from build123d import *

# Parameters (mm, degrees)
F0_R     = 11.509137
F1_DEPTH = 25.4
F2_DEPTH = 50.8


with BuildPart() as f1:
    # F0 (on Front) → F1 (new body)
    with BuildSketch(Plane.XZ):
        with BuildLine():
            ThreePointArc((-23.485197, 0), (0, -23.485197), (23.485197, 0))
            ThreePointArc((23.485197, 0), (0, 23.485197), (-23.485197, 0))
        make_face()
        Circle(F0_R, mode=Mode.SUBTRACT)
        with BuildLine():
            ThreePointArc((-23.485197, 0), (0, 23.485197), (23.485197, 0))
            Line((23.485197, 0), (23.485197, 74.391678))
            ThreePointArc((23.485197, 74.391678), (0, 50.906481), (-23.485197, 74.391678))
            Line((-23.485197, 74.391678), (-23.485197, 0))
        make_face()
        with BuildLine():
            ThreePointArc((-23.485197, 74.391678), (0, 50.906481), (23.485197, 74.391678))
            ThreePointArc((23.485197, 74.391678), (0, 97.876875), (-23.485197, 74.391678))
        make_face()
        with Locations((0, 74.391678)):
            Circle(F0_R, mode=Mode.SUBTRACT)
    extrude(amount=F1_DEPTH)

    # F0 (on Front) → F2 (join)
    with BuildSketch(Plane.XZ):
        with BuildLine():
            ThreePointArc((-23.485197, 0), (0, -23.485197), (23.485197, 0))
            ThreePointArc((23.485197, 0), (0, 23.485197), (-23.485197, 0))
        make_face()
        Circle(F0_R, mode=Mode.SUBTRACT)
    extrude(amount=-F2_DEPTH)

    # F3: F1 across face


with BuildPart() as f1_1:
    add(f1.part)
    add(f1.part.mirror(Plane(origin=(0, 50.8, 0), x_dir=(1, 0, 0), z_dir=(0, 1, 0))))


solid = f1_1.part
Source: CAD feature listing. Evaluate the final solid. Frame: model axes, mm. Coordinates: 2 decimals unless noted, no trailing zeros. Loops run counter-clockwise (first coordinate to the right, second up) from the corner with the lowest first, then second, coordinate; pieces in that order, holes last. Notation, with made-up numbers: (73.25, 37) - (97.25, 37) arc R38 cw to (97.25, 75) - close; hole circle Ø7 at (-17, 68). An arc over 180 degrees is marked (long way). One line per question, with ' | ' between items.
1) First-contact query: P1, Ø10, axis at y = 29.5, z = 31.5, coming from the +X side; P2, Ø5, axis at x = -0.5, y = 67, coming from the +Z side; P3, Ø3, axis at x = -13, y = 55, coming from the +Z side; P4, Ø10, axis at x = 13, y = -1.5, coming from the +Z side. Flat tips, straight axial feed; report the tip coordinate or a pass-through.
Report:
P1: passes through | P2: stops at z = 23.49 | P3: stops at z = 20.48 | P4: stops at z = 96.47
2) Pull-direction query (Y, two-part tool) for faces 1 (the face through (0.52, 114.12, 97.87)), 2 (the face through (0, -25.4, 38)), 3 (the face through (0, 0, 50)); classes: released by +Y, released by -Y, zero draft, split by the parting line, or undercut.
Report:
face 1: zero draft | face 2: released by -Y | face 3: undercut
3) Section C-C, the plane y = -4. Return loops of the section in (x, z), then the cut area to 3 significant figures.
Report:
outline: (-23.49, 0) arc R23.49 ccw to (23.49, 0) - (23.49, 74.39) arc R23.49 ccw to (-23.49, 74.39) - close; hole circle Ø23.02 at (0, 0); hole circle Ø23.02 at (0, 74.39) | area: 4,390 mm²
4) Section B-B, the plane z = 39. Return loops of the section in (x, y).
Report:
outline: (-23.49, -25.4) - (23.49, -25.4) - (23.49, 0) - (-23.49, 0) - close; (-23.49, 101.6) - (23.49, 101.6) - (23.49, 127) - (-23.49, 127) - close
5) Section D-D, the plane z = 69.5. Return loops of the section in (x, y), then the cut area to 3 significant figures.
Report:
outline: (-23.49, -25.4) - (-10.42, -25.4) - (-10.42, 0) - (-23.49, 0) - close; (-23.49, 101.6) - (-10.42, 101.6) - (-10.42, 127) - (-23.49, 127) - close; (10.42, -25.4) - (23.49, -25.4) - (23.49, 0) - (10.42, 0) - close; (10.42, 101.6) - (23.49, 101.6) - (23.49, 127) - (10.42, 127) - close | area: 1,330 mm²
6) Section A-A, the plane x = 0. Return loops of the section in (y, z).
Report:
outline: (-25.4, -23.49) - (127, -23.49) - (127, -11.51) - (-25.4, -11.51) - close; (-25.4, 11.51) - (127, 11.51) - (127, 62.88) - (101.6, 62.88) - (101.6, 23.49) - (0, 23.49) - (0, 62.88) - (-25.4, 62.88) - close; (-25.4, 85.9) - (0, 85.9) - (0, 97.88) - (-25.4, 97.88) - close; (101.6, 85.9) - (127, 85.9) - (127, 97.88) - (101.6, 97.88) - close
7) Line query: line 1 along Z through (x, y) = (0, 120.25); line 2 along Y through (x, z) = (-11.5, 90.5); line 3 along Z through (x, y) = (0, 25.5). Output: solid intervals per line, ascending.
Report:
line 1: z = -23.49 to -11.51, 11.51 to 62.88, 85.9 to 97.88 | line 2: y = -25.4 to 0, 101.6 to 127 | line 3: z = -23.49 to -11.51, 11.51 to 23.49
